Can you work these out from the drawing? Everything is in mm from the part's minimum corner. A direction names the side the tool comes from. Coordinates: 2 decimals unless noted, no trailing zeros. Loops run counter-clockwise (first coordinate to the right, second up) from the corner with the lowest first, then second, coordinate; pieces in that order, holes last. Notation, with made-up numbers: (17.5, 56) - (47.5, 56) arc R9 cw to (47.5, 71) - close; hole circle Ø1 at (38.5, 88). An arc over 180 degrees is marked (long way). Put each result on its own line as item: value. Start each with the question number.
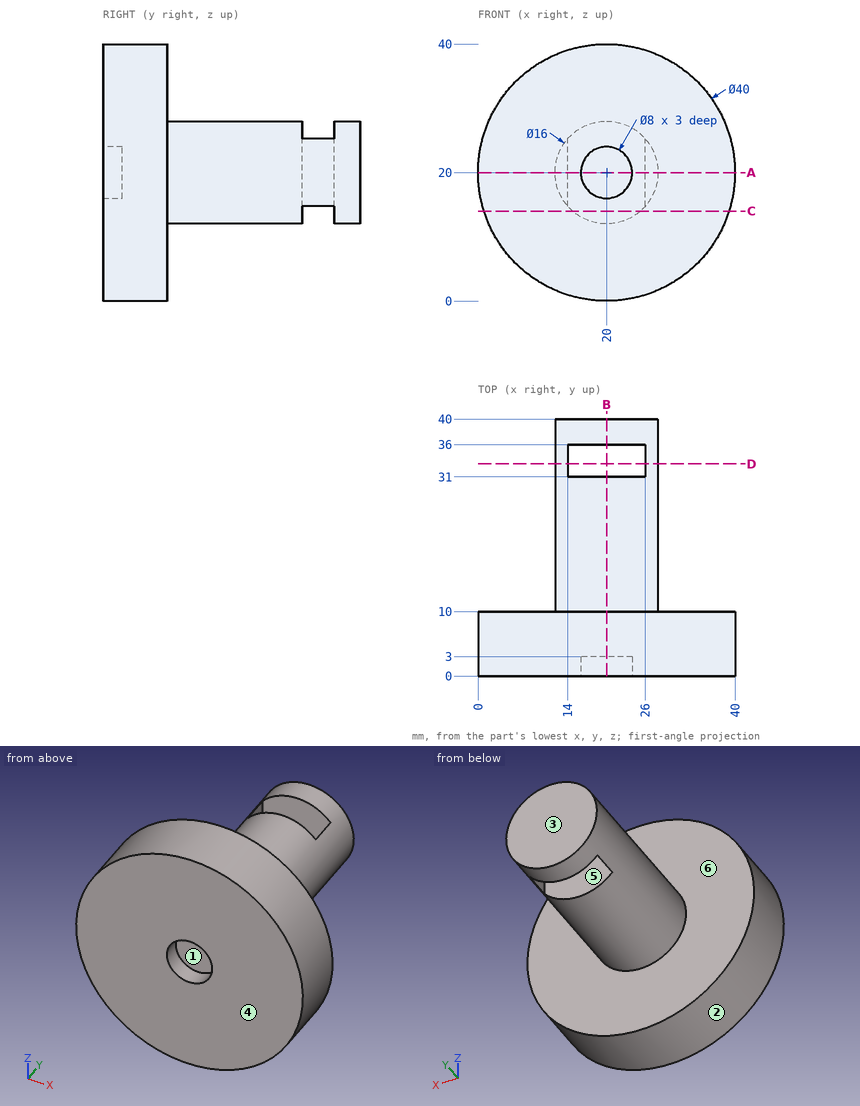
Q1. On a 3-axis mill with a long thin cutter (end or side, diameter ignored), from which of +Z, -Z, +X, -X, +Y, -Y can I reach the whole of each face in a straight line? I mean the marked faces 4, 5 and 6. Say none if no direction works.
Q2. I want a section at C-C on z = 14. List the corners of the cut face in (x, y) for me.
Q3. I want a section at A-A on z = 20. List the corners of the cut face in (x, y) for me, and give its area (3 significant figures).
Q4. I want a section at D-D on y = 33. List the corners of the cut face in (x, z) for me, and give its area (3 significant figures).
Q5. Will these pins go through, and if not, where does the flat tip stop? pin 1 (10 mm diameter, centred on y = 19, z = 16, fed in from +X); pin 2 (2 mm diameter, centred on y = 10.5, z = 4.5, fed in from +X); pin 3 (12 mm diameter, centred on y = 8.5, z = 12.5, fed in from +X).
Q6. Please list where these lines run through material, in increasing order: line 1 along X through (y, z) = (1.4, 20); line 2 along Y through (x, z) = (23, 17); line 3 along Y through (x, z) = (6, 32.5). Write a range as [from, to].
Q7. I want a section at B-B on x = 20. List the corners of the cut face in (y, z) for me, and give its area (3 significant figures).
Q8. We'd pull the mould along Z, two halves only. Please class the marked faces 1, 2 and 3: released by +Z, released by -Z, zero draft, split by the parting line, or undercut.
Calculated:
1. face 4: +Z, -Z, +X, -X, -Y
1. face 5: +Z, -Z
1. face 6: +Y
2. outline: (0.92, 0) - (39.08, 0) - (39.08, 10) - (25.29, 10) - (25.29, 31) - (14.71, 31) - (14.71, 10) - (0.92, 10) - close; (14.71, 36) - (25.29, 36) - (25.29, 40) - (14.71, 40) - close
3. outline: (0, 0) - (16, 0) - (16, 3) - (24, 3) - (24, 0) - (40, 0) - (40, 10) - (28, 10) - (28, 40) - (12, 40) - (12, 10) - (0, 10) - close; hole (14, 31) - (26, 31) - (26, 36) - (14, 36) - close
3. area: 796 mm2
4. outline: (14, 14.71) - (14, 25.29) arc R8 ccw to start; (26, 14.71) arc R8 ccw to (26, 25.29) - close
4. area: 29.0 mm2
5. pin 1: x = 28
5. pin 2: x = 33.63
5. pin 3: x = 39.94
6. line 1: [0, 16], [24, 40]
6. line 2: [0, 31], [36, 40]
6. line 3: [0, 10]
7. outline: (0, 0) - (10, 0) - (10, 12) - (31, 12) - (31, 28) - (10, 28) - (10, 40) - (0, 40) - (0, 24) - (3, 24) - (3, 16) - (0, 16) - close; (36, 12) - (40, 12) - (40, 28) - (36, 28) - close
7. area: 776 mm2
8. face 1: undercut
8. face 2: split by the parting line
8. face 3: zero draft
